```python
from build123d import *

# Parameters (mm, degrees)
SKETCH1_R           = 14
BOSS_EXTRUDE1_DEPTH = 15
BOSS_EXTRUDE2_DEPTH = 6.9
BOSS_EXTRUDE3_DEPTH = 15
SKETCH4_R           = 4.1
CUT_EXTRUDE1_DEPTH  = 42.876126850509955


with BuildPart() as part:
    # Sketch1 → Boss-Extrude1 (new body)
    with BuildSketch(Plane.XY):
        Circle(SKETCH1_R)
    extrude(amount=BOSS_EXTRUDE1_DEPTH)

    # Sketch2 → Boss-Extrude2 (add)
    with BuildSketch(Plane.XY.offset(15)):
        with BuildLine():
            Line((-6.600000000000001, 3.810511776651534), (-6.600000000000002, 12.34665946724052))
            ThreePointArc((-6.600000000000002, 12.34665946724052), (-2.57e-15, -14), (6.599999999999997, 12.34665946724052))
            Line((6.599999999999997, 12.34665946724052), (6.599999999999997, 3.695041722813614))
            Line((6.599999999999997, 3.695041722813614), (6.599999999999998, -3.810511776651528))
            Line((6.599999999999998, -3.810511776651528), (-1.31e-15, -7.62102355330306))
            Line((-1.31e-15, -7.62102355330306), (-6.600000000000001, -3.8105117766515293))
            Line((-6.600000000000001, -3.8105117766515293), (-6.600000000000001, 3.810511776651534))
        make_face()
    extrude(amount=BOSS_EXTRUDE2_DEPTH)

    # Sketch3 → Boss-Extrude3 (add)
    with BuildSketch(Plane.XY.offset(21.9)):
        with BuildLine():
            ThreePointArc((6.599999999999995, 12.346659467240523), (-2.25e-15, 13.999999999999998), (-6.600000000000002, 12.34665946724052))
            ThreePointArc((-6.600000000000002, 12.34665946724052), (-2.57e-15, -14), (6.599999999999995, 12.346659467240523))
        make_face()
    extrude(amount=BOSS_EXTRUDE3_DEPTH)

    # Sketch4 → Cut-Extrude1 (cut, through all)
    with BuildSketch(Plane.XY.offset(36.900000000000006)):
        Circle(SKETCH4_R)
    extrude(amount=-CUT_EXTRUDE1_DEPTH, mode=Mode.SUBTRACT)

    # Chamfer1
    # the kernel refuses this chamfer: 0.5 mm, written as the material it takes off along each edge
    with BuildSketch(Plane(origin=(0, 0, 0), x_dir=(1, 0, 0), z_dir=(0, -1, 0))) as chamfer1_piece_1:
        with BuildLine():
            Line((14.01414213562373, 0.5141421356237309), (13.48585786437627, -0.01414213562373095))
            Line((13.48585786437627, -0.01414213562373095), (13.48585786437627, -0.02414213562373095))
            ThreePointArc((13.48585786437627, -0.02414213562373095), (13.742928932188136, -0.01), (14, -0.01))
            Line((14, -0.01), (14.01, 0))
            ThreePointArc((14.01, 0), (14.01, 0.25707106781186545), (14.02414213562373, 0.5141421356237309))
            Line((14.02414213562373, 0.5141421356237309), (14.01414213562373, 0.5141421356237309))
        make_face()
    revolve(axis=Axis((0, 0, 0), (0, 0, 1)), mode=Mode.SUBTRACT)
    with BuildSketch(Plane(origin=(1.11e-15, 1.7e-16, 36.9), x_dir=(0.4714285714285716, 0.8819042476600372, 0), z_dir=(-0.8819042476600372, 0.4714285714285716, 0))) as chamfer1_piece_2:
        with BuildLine():
            Line((14.01414213562373, 0.5141421356237288), (13.48585786437627, -0.01414213562372879))
            Line((13.48585786437627, -0.01414213562372879), (13.48585786437627, -0.0241421356237268))
            ThreePointArc((13.48585786437627, -0.0241421356237268), (13.742928932188134, -0.00999999999999801), (14, -0.00999999999999801))
            Line((14, -0.00999999999999801), (14.01, 0))
            ThreePointArc((14.01, 0), (14.01, 0.2570710678118644), (14.02414213562373, 0.5141421356237288))
            Line((14.02414213562373, 0.5141421356237288), (14.01414213562373, 0.5141421356237288))
        make_face()
    revolve(axis=Axis((1.11e-15, 1.7e-16, 36.9), (0, 0, -1)), mode=Mode.SUBTRACT)
    with BuildSketch(Plane(origin=(0, 0, 0), x_dir=(1, 0, 0), z_dir=(0, -1, 0))) as chamfer1_piece_3:
        with BuildLine():
            Line((4.61414213562373, -0.01414213562373095), (4.085857864376269, 0.5141421356237309))
            Line((4.085857864376269, 0.5141421356237309), (4.075857864376269, 0.5141421356237309))
            ThreePointArc((4.075857864376269, 0.5141421356237309), (4.09, 0.2570710678118644), (4.09, 0))
            Line((4.09, 0), (4.1, -0.01))
            ThreePointArc((4.1, -0.01), (4.357071067811865, -0.01), (4.61414213562373, -0.02414213562373095))
            Line((4.61414213562373, -0.02414213562373095), (4.61414213562373, -0.01414213562373095))
        make_face()
    revolve(axis=Axis((0, 0, 0), (0, 0, 1)), mode=Mode.SUBTRACT)
    with BuildSketch(Plane(origin=(0, 0, 36.900000000000006), x_dir=(1, 0, 0), z_dir=(0, -1, 0))) as chamfer1_piece_4:
        with BuildLine():
            Line((4.614142135623731, 0.01414213562372169), (4.085857864376268, -0.5141421356237288))
            Line((4.085857864376268, -0.5141421356237288), (4.075857864376268, -0.5141421356237288))
            ThreePointArc((4.075857864376268, -0.5141421356237288), (4.09, -0.2570710678118644), (4.09, 0))
            Line((4.09, 0), (4.1, 0.00999999999999801))
            ThreePointArc((4.1, 0.00999999999999801), (4.357071067811866, 0.00999999999999091), (4.614142135623731, 0.0241421356237197))
            Line((4.614142135623731, 0.0241421356237197), (4.614142135623731, 0.01414213562372169))
        make_face()
    revolve(axis=Axis((0, 0, 36.900000000000006), (0, 0, 1)), mode=Mode.SUBTRACT)


solid = part.part
```
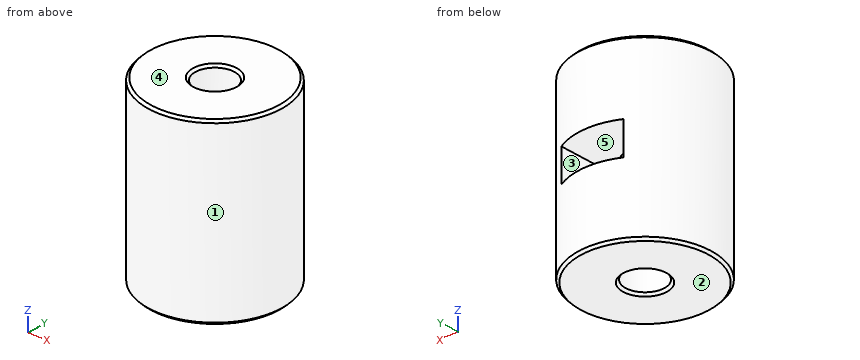
Input: part model. Units: mm. Frame: model coordinates. Face numbers are marked on the shaded views. A direction names the side the tool comes from. Coordinates: 2 decimals unless noted, no trailing zeros. Loops run counter-clockwise (first coordinate to the right, second up) from the corner with the lowest first, then second, coordinate; pieces in that order, holes last. Notation, with made-up numbers: M 81,21 L 106,21 A22 ccw 106,28 Z; hole C 27,-13 d5. An arc over 180 degrees is marked long. Use a Markdown table: item, result. Add a question column.
1) Line query: L1, parallel to Y at x = 0, z = 4.75; L2, parallel to Z at x = -2.5, y = -4.5; L3, parallel to X at y = -0.5, z = 13.5. Output: solid intervals per line, ascending. Write a range as from..to.
2) Pin query (flat end, axial travel): P1, Ø3.5, axis at y = 5.5, z = 17.5, coming from the -X side; P2, Ø8, axis at y = 10.5, z = 9.5, coming from the +X side; P3, Ø3, axis at x = 6.5, z = 20, coming from the +Y side. Return the tip coordinate at first contact, or that it passes through.
3) Section A-A, the plane z = 3. Return the cut outline in (x, y).
4) Draft query along X for the marked faces 1, 2 and 3. Return one class per face: +X half, -X half, draft (parallel to the pull), parting line (faces both ways), or undercut.
5) Section B-B, the plane z = 19. Return the cut outline in (x, y).
6) Set-up query: the marked faces 4 and 5. Return all of +Z, -Z, +X, -X, +Y, -Y with unobstructed straight access to the full face (end or side cutting, diameter ignored); none if empty.
Answer below:
| question | item | result |
|---|---|---|
| 1 | L1 | -14..-4.1, 4.1..14 |
| 1 | L2 | 0..15, 21.9..36.9 |
| 1 | L3 | -13.99..-4.07, 4.07..13.99 |
| 2 | P1 | x = -13.49 |
| 2 | P2 | x = 12.4 |
| 2 | P3 | y = 12.35 |
| 3 | outline | C 0,0 d28; hole C 0,0 d8.2 |
| 4 | face 1 | parting line |
| 4 | face 2 | draft |
| 4 | face 3 | undercut |
| 5 | outline | M -6.6,-3.81 L -6.6,12.35 A14 ccw long 6.6,12.35 L 6.6,-3.81 L 0,-7.62 Z |
| 6 | face 4 | +Z, +X, -X, +Y, -Y |
| 6 | face 5 | +Y |
